Can you work these out from the model? Positions are in its coordinate system, mm. Face numbers are marked on the shaded views. A direction names the side the tool comes from. Coordinates: 2 decimals unless noted, no trailing zeros. Loops run counter-clockwise (first coordinate to the right, second up) from the corner with the lowest first, then second, coordinate; pieces in that order, holes last.
```python
from build123d import *

# Parameters (mm, degrees)
SKETCH1_W            = 100
SKETCH1_H            = 85
BASE_FLANGE1_DEPTH   = 2
EDGE_FLANGE2_DEPTH   = 100
EDGE_FLANGE2_2_DEPTH = 100
SKETCH16_R           = 1.5
SKETCH16_W           = 20
SKETCH16_H           = 42
CUT_EXTRUDE2_DEPTH   = 2
SKETCH18_R           = 1.5
CUT_EXTRUDE3_DEPTH   = 10
SKETCH19_R           = 1.5
CUT_EXTRUDE5_DEPTH   = 10
CUT_EXTRUDE6_DEPTH   = 10
SKETCH21_R           = 1.5
CUT_EXTRUDE7_DEPTH   = 10


# Read off the part's stored shape, not the designer's step: Edge-Flange2
# Sheet-metal steps are written as plain solids
with BuildPart() as part:
    # Sketch1 → Base-Flange1 (new body)
    with BuildSketch(Plane(origin=(0, 0, 0), x_dir=(1, 0, 0), z_dir=(0, 1, 0))):
        with Locations((50, 42.5)):
            Rectangle(SKETCH1_W, SKETCH1_H)
    extrude(amount=-BASE_FLANGE1_DEPTH)

    # Edge-Flange2 outline → Edge-Flange2 (cut)
    with BuildSketch(Plane.YZ):
        with BuildLine():
            Line((-2, 0), (-1.3683, -0.364712165))
            ThreePointArc((-1.3683, -0.364712165), (-0.36663488, -1.366377285), (0, -2.734677285))
            Line((0, -2.734677285), (0, 0))
            Line((0, 0), (-2, 0))
        make_face()
    extrude(amount=EDGE_FLANGE2_DEPTH, mode=Mode.SUBTRACT)

    # Edge-Flange2 2 outline → Edge-Flange2 2 (add)
    with BuildSketch(Plane.YZ):
        with BuildLine():
            Line((-2, -2.734677285), (-2, 0))
            Line((-2, 0), (-13.856406461, 6.845299462))
            Line((-13.856406461, 6.845299462), (-14.856406461, 5.113248654))
            Line((-14.856406461, 5.113248654), (-2.3683, -2.096762973))
            ThreePointArc((-2.3683, -2.096762973), (-2.098685688, -2.366377285), (-2, -2.734677285))
        make_face()
    extrude(amount=EDGE_FLANGE2_2_DEPTH)

    # Sketch16 → Cut-Extrude2 (cut)
    with BuildSketch(Plane(origin=(0, 0, 0), x_dir=(1, 0, 0), z_dir=(0, 1, 0))):
        with Locations(Location((5, 8, 0), (0, 0, 270))):
            Circle(SKETCH16_R)
        with Locations(Location((50, 80, 0), (0, 0, 270))):
            Circle(SKETCH16_R)
        with Locations(Location((5, 40.5, 0), (0, 0, 270))):
            Circle(SKETCH16_R)
        with Locations(Location((95, 8, 0), (0, 0, 90))):
            Circle(SKETCH16_R)
        with Locations(Location((95, 40.5, 0), (0, 0, 90))):
            Circle(SKETCH16_R)
        with Locations(Location((25, 73, 0), (0, 0, 270))):
            Circle(SKETCH16_R)
        with Locations(Location((25, 55, 0), (0, 0, 90))):
            Circle(SKETCH16_R)
        with Locations(Location((75, 55, 0), (0, 0, 270))):
            Circle(SKETCH16_R)
        with Locations(Location((75, 73, 0), (0, 0, 90))):
            Circle(SKETCH16_R)
        with Locations((10, 64)):
            Rectangle(SKETCH16_W, SKETCH16_H)
        with Locations((90, 64)):
            Rectangle(SKETCH16_W, SKETCH16_H)
    extrude(amount=-CUT_EXTRUDE2_DEPTH, mode=Mode.SUBTRACT)

    # Sketch18 → Cut-Extrude3 (cut)
    with BuildSketch(Plane(origin=(0, 0, 0), x_dir=(1, 0, 0), z_dir=(0, 1, 0))):
        with Locations(Location((22, 8, 0), (0, 0, 270))):
            Circle(SKETCH18_R)
        with Locations(Location((78, 8, 0), (0, 0, 90))):
            Circle(SKETCH18_R)
    extrude(amount=-CUT_EXTRUDE3_DEPTH, mode=Mode.SUBTRACT)

    # Sketch19 → Cut-Extrude5 (cut)
    with BuildSketch(Plane(origin=(0, 0, 0), x_dir=(1, 0, 0), z_dir=(0, 1, 0))):
        with Locations(Location((30, 6.646195809, 0), (0, 0, 270))):
            Circle(SKETCH19_R)
        with Locations(Location((30, 10.646195809, 0), (0, 0, 270))):
            Circle(SKETCH19_R)
        with Locations(Location((70, 6.646195809, 0), (0, 0, 90))):
            Circle(SKETCH19_R)
        with Locations(Location((70, 10.646195809, 0), (0, 0, 90))):
            Circle(SKETCH19_R)
    extrude(amount=-CUT_EXTRUDE5_DEPTH, mode=Mode.SUBTRACT)

    # Sketch20 → Cut-Extrude6 (cut)
    with BuildSketch(Plane(origin=(0, 0, 0), x_dir=(1, 0, 0), z_dir=(0, 1, 0))):
        with BuildLine():
            Line((59.619346947, 49.788219715), (66.548820549, 49.788219715))
            ThreePointArc((66.548820549, 49.788219715), (67.25592733, 49.495326496), (67.548820549, 48.788219715))
            Line((67.548820549, 48.788219715), (67.548820549, 47.788219715))
            ThreePointArc((67.548820549, 47.788219715), (67.25592733, 47.081112934), (66.548820549, 46.788219715))
            Line((66.548820549, 46.788219715), (59.619346947, 46.788219715))
            ThreePointArc((59.619346947, 46.788219715), (58.912240166, 47.081112934), (58.619346947, 47.788219715))
            Line((58.619346947, 47.788219715), (58.619346947, 48.788219715))
            ThreePointArc((58.619346947, 48.788219715), (58.912240166, 49.495326496), (59.619346947, 49.788219715))
        make_face()
        with BuildLine():
            Line((30.883992336, 20.788219715), (37.619346947, 20.788219715))
            ThreePointArc((37.619346947, 20.788219715), (38.326453728, 20.495326496), (38.619346947, 19.788219715))
            Line((38.619346947, 19.788219715), (38.619346947, 18.788219715))
            ThreePointArc((38.619346947, 18.788219715), (38.326453728, 18.081112934), (37.619346947, 17.788219715))
            Line((37.619346947, 17.788219715), (30.883992336, 17.788219715))
            ThreePointArc((30.883992336, 17.788219715), (30.176885554, 18.081112934), (29.883992336, 18.788219715))
            Line((29.883992336, 18.788219715), (29.883992336, 19.788219715))
            ThreePointArc((29.883992336, 19.788219715), (30.176885554, 20.495326496), (30.883992336, 20.788219715))
        make_face()
        with BuildLine():
            Line((59.619346947, 20.788219715), (66.548820549, 20.788219715))
            ThreePointArc((66.548820549, 20.788219715), (67.25592733, 20.495326496), (67.548820549, 19.788219715))
            Line((67.548820549, 19.788219715), (67.548820549, 18.788219715))
            ThreePointArc((67.548820549, 18.788219715), (67.25592733, 18.081112934), (66.548820549, 17.788219715))
            Line((66.548820549, 17.788219715), (59.619346947, 17.788219715))
            ThreePointArc((59.619346947, 17.788219715), (58.912240166, 18.081112934), (58.619346947, 18.788219715))
            Line((58.619346947, 18.788219715), (58.619346947, 19.788219715))
            ThreePointArc((58.619346947, 19.788219715), (58.912240166, 20.495326496), (59.619346947, 20.788219715))
        make_face()
        with BuildLine():
            Line((30.883992336, 49.788219715), (37.619346947, 49.788219715))
            ThreePointArc((37.619346947, 49.788219715), (38.326453728, 49.495326496), (38.619346947, 48.788219715))
            Line((38.619346947, 48.788219715), (38.619346947, 47.788219715))
            ThreePointArc((38.619346947, 47.788219715), (38.326453728, 47.081112934), (37.619346947, 46.788219715))
            Line((37.619346947, 46.788219715), (30.883992336, 46.788219715))
            ThreePointArc((30.883992336, 46.788219715), (30.176885554, 47.081112934), (29.883992336, 47.788219715))
            Line((29.883992336, 47.788219715), (29.883992336, 48.788219715))
            ThreePointArc((29.883992336, 48.788219715), (30.176885554, 49.495326496), (30.883992336, 49.788219715))
        make_face()
    extrude(amount=-CUT_EXTRUDE6_DEPTH, mode=Mode.SUBTRACT)

    # Sketch21 → Cut-Extrude7 (cut)
    with BuildSketch(Plane(origin=(0, 0, 0), x_dir=(1, 0, 0), z_dir=(0, 1, 0))):
        with Locations(Location((26, 82, 0), (0, 0, 270))):
            Circle(SKETCH21_R)
        with Locations(Location((30, 82, 0), (0, 0, 270))):
            Circle(SKETCH21_R)
        with Locations(Location((74, 82, 0), (0, 0, 90))):
            Circle(SKETCH21_R)
        with Locations(Location((70, 82, 0), (0, 0, 90))):
            Circle(SKETCH21_R)
        with BuildLine():
            Line((54, 51), (53, 51))
            ThreePointArc((53, 51), (52.292893219, 51.292893219), (52, 52))
            Line((52, 52), (52, 53))
            ThreePointArc((52, 53), (52.292893219, 53.707106781), (53, 54))
            Line((53, 54), (54, 54))
            ThreePointArc((54, 54), (54.707106781, 53.707106781), (55, 53))
            Line((55, 53), (55, 52))
            ThreePointArc((55, 52), (54.707106781, 51.292893219), (54, 51))
        make_face()
        with BuildLine():
            Line((46, 77), (47, 77))
            ThreePointArc((47, 77), (47.707106781, 76.707106781), (48, 76))
            Line((48, 76), (48, 75))
            ThreePointArc((48, 75), (47.707106781, 74.292893219), (47, 74))
            Line((47, 74), (46, 74))
            ThreePointArc((46, 74), (45.292893219, 74.292893219), (45, 75))
            Line((45, 75), (45, 76))
            ThreePointArc((45, 76), (45.292893219, 76.707106781), (46, 77))
        make_face()
        with BuildLine():
            Line((46, 54), (47, 54))
            ThreePointArc((47, 54), (47.707106781, 53.707106781), (48, 53))
            Line((48, 53), (48, 52))
            ThreePointArc((48, 52), (47.707106781, 51.292893219), (47, 51))
            Line((47, 51), (46, 51))
            ThreePointArc((46, 51), (45.292893219, 51.292893219), (45, 52))
            Line((45, 52), (45, 53))
            ThreePointArc((45, 53), (45.292893219, 53.707106781), (46, 54))
        make_face()
        with BuildLine():
            Line((54, 74), (53, 74))
            ThreePointArc((53, 74), (52.292893219, 74.292893219), (52, 75))
            Line((52, 75), (52, 76))
            ThreePointArc((52, 76), (52.292893219, 76.707106781), (53, 77))
            Line((53, 77), (54, 77))
            ThreePointArc((54, 77), (54.707106781, 76.707106781), (55, 76))
            Line((55, 76), (55, 75))
            ThreePointArc((55, 75), (54.707106781, 74.292893219), (54, 74))
        make_face()
    extrude(amount=-CUT_EXTRUDE7_DEPTH, mode=Mode.SUBTRACT)


solid = part.part
```
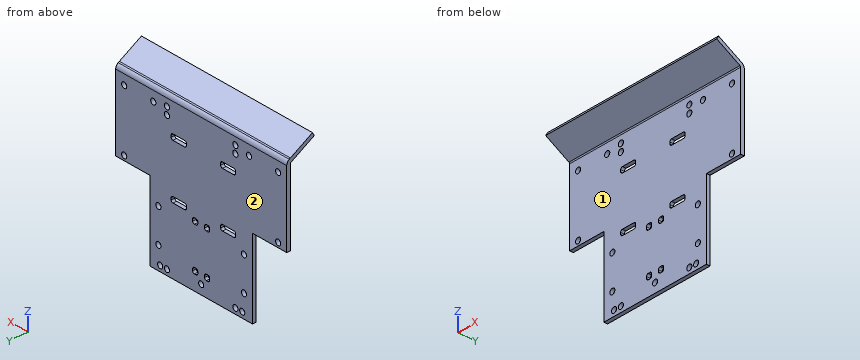
Item 1: I need wall thicknesses on line 1 along X through (y, z) = (-0.65, -82); line 2 along X through (y, z) = (-0.8, -40.5); line 3 along X through (y, z) = (-1.5, -73). Which ranges of each line are inside material? Lowest first, please.
Results are:
line 1: x = 20 to 24.5, 27.5 to 28.5, 31.5 to 68.5, 71.5 to 72.5, 75.5 to 80
line 2: x = 0 to 3.5, 6.5 to 93.5, 96.5 to 100
line 3: x = 20 to 23.5, 26.5 to 73.5, 76.5 to 80
Item 2: I'm going to push flat-ended pins straight in: P1, Ø4, axis at y = -4.5, z = -63.5, coming from the -X side; P2, Ø4, axis at x = 70, z = -10.65, coming from the -Y side; P3, Ø2, axis at x = 7.5, y = -0.5, coming from the -Z side; P4, Ø0.5, axis at y = -1, z = -75.5, coming from the -X side. Where does each tip first touch, or does it pass through?
Results are:
P1: passes through
P2: stops at y = -2
P3: stops at z = -43
P4: stops at x = 20
Item 3: On a 3-axis mill with a long thin cutter (end or side, diameter ignored), from which of +Z, -Z, +X, -X, +Y, -Y can I reach the whole of each face in a straight line? I mean the marked faces 1 and 2. Say none if no direction works.
Results are:
face 1: -Z, +X, -X, -Y
face 2: +Z, -Z, +X, -X, +Y
Item 4: Suppose I cut it at C-C, the plane x = 22. Please give me the cut outline in (y, z).
Results are:
outline: (-14.86, 5.11) - (-2.37, -2.1) arc R0.74 cw to (-2, -2.73) - (-2, -6.5) - (0, -6.5) - (0, -2.73) arc R2.74 ccw to (-1.37, -0.36) - (-13.86, 6.85) - close; (-2, -85) - (0, -85) - (0, -9.5) - (-2, -9.5) - close
Item 5: Suppose I cut it at A-A, the plane x = 34. Please give me the cut outline in (y, z), plus the area to 3 significant figures.
Results are:
outline: (-14.86, 5.11) - (-2.37, -2.1) arc R0.74 cw to (-2, -2.73) - (-2, -17.79) - (0, -17.79) - (0, -2.73) arc R2.74 ccw to (-1.37, -0.36) - (-13.86, 6.85) - close; (-2, -85) - (0, -85) - (0, -49.79) - (-2, -49.79) - close; (-2, -46.79) - (0, -46.79) - (0, -20.79) - (-2, -20.79) - close
area: 185 mm2
Item 6: Suppose I cut it at B-B, the plane x = 70. Please give me the cut outline in (y, z).
Results are:
outline: (-14.86, 5.11) - (-2.37, -2.1) arc R0.74 cw to (-2, -2.73) - (-2, -5.15) - (0, -5.15) - (0, -2.73) arc R2.74 ccw to (-1.37, -0.36) - (-13.86, 6.85) - close; (-2, -85) - (0, -85) - (0, -83.5) - (-2, -83.5) - close; (-2, -80.5) - (0, -80.5) - (0, -12.15) - (-2, -12.15) - close; (-2, -9.15) - (0, -9.15) - (0, -8.15) - (-2, -8.15) - close
Item 7: Suppose I cut it at D-D, the plane z = -25. Please give me the cut outline in (x, y), plus the area to 3 significant figures.
Results are:
outline: (0, -2) - (100, -2) - (100, 0) - (0, 0) - close
area: 200 mm2
